Could you check a few things on this model? Use its own coordinates, in mm. A direction names the side the tool comes from. Give positions to 0.01 mm unless a question says otherwise; leave off trailing zeros. Write each loop counter-clockwise with the first axis right and the second up, starting at its lowest first coordinate (ties: lowest second). Pieces come first, ordered by that corner, then holes. Notation, with made-up numbers: M -10,-16.5 L 8,-16.5 A15 cw 8,7.5 Z; hole C 69.25,79.25 d7. An arc over 180 degrees is marked long. Answer as a JSON object with one key per item and string values. Group by question number.
```python
from build123d import *

# Parameters (mm, degrees)
F1_DEPTH    = 7.62
F2_T1_DEPTH = 231.4037837241


# Not quite as in the source:
# - a fillet or chamfer that OpenCascade refuses, or shapes differently, is made with other operations: its cross-section is extruded or revolved along the edge and cut away or added


with BuildPart() as f1:
    # F0 (on Top) → F1 (new body)
    with BuildSketch(Plane.XY):
        with BuildLine():
            ThreePointArc((64.7411976721, 47.7861853946), (-11.4588023279, 55.4061853946), (-87.6588023279, 47.7861853946))
            Line((-87.6588023279, 47.7861853946), (64.7411976721, 47.7861853946))
        make_face()
        with BuildLine():
            Line((-87.6588023279, -28.4138146054), (-87.6588023279, 47.7861853946))
            ThreePointArc((-87.6588023279, 47.7861853946), (-102.8988023279, 9.6861853946), (-87.6588023279, -28.4138146054))
        make_face()
        with BuildLine():
            Line((64.7411976721, 47.7861853946), (-87.6588023279, 47.7861853946))
            Line((-87.6588023279, 47.7861853946), (-87.6588023279, -28.4138146054))
            Line((-87.6588023279, -28.4138146054), (64.7411976721, -28.4138146054))
            ThreePointArc((64.7411976721, -28.4138146054), (58.4381171141, -26.858273051), (52.536175044, -24.1535339048))
            ThreePointArc((52.536175044, -24.1535339048), (51.7671122609, -23.7311786415), (51.0407896557, -23.2389419038))
            ThreePointArc((51.0407896557, -23.2389419038), (46.5861857996, -19.8140652327), (42.744152416, -15.7138146054))
            ThreePointArc((42.744152416, -15.7138146054), (46.5861857996, -11.6135639782), (51.0407896557, -8.188687307))
            ThreePointArc((51.0407896557, -8.188687307), (51.7671122609, -7.6964505693), (52.536175044, -7.2740953061))
            ThreePointArc((52.536175044, -7.2740953061), (58.4381171141, -4.5693561598), (64.7411976721, -3.0138146054))
            Line((64.7411976721, -3.0138146054), (64.7411976721, 22.3861853946))
            ThreePointArc((64.7411976721, 22.3861853946), (58.4381171141, 23.941726949), (52.536175044, 26.6464660952))
            ThreePointArc((52.536175044, 26.6464660952), (51.7671122609, 27.0688213585), (51.0407896557, 27.5610580962))
            ThreePointArc((51.0407896557, 27.5610580962), (46.5861857996, 30.9859347673), (42.744152416, 35.0861853946))
            ThreePointArc((42.744152416, 35.0861853946), (46.5861857996, 39.1864360218), (51.0407896557, 42.611312693))
            ThreePointArc((51.0407896557, 42.611312693), (51.7671122609, 43.1035494307), (52.536175044, 43.5259046939))
            ThreePointArc((52.536175044, 43.5259046939), (58.4381171141, 46.2306438402), (64.7411976721, 47.7861853946))
        make_face()
        with BuildLine():
            Line((64.7411976721, -28.4138146054), (-87.6588023279, -28.4138146054))
            ThreePointArc((-87.6588023279, -28.4138146054), (-11.4588023279, -36.0338146054), (64.7411976721, -28.4138146054))
        make_face()
        with BuildLine():
            ThreePointArc((51.0407896557, -23.2389419038), (49.0199759717, -21.171856557), (47.7230187251, -18.5883644093))
            Line((47.7230187251, -18.5883644093), (42.744152416, -15.7138146054))
            ThreePointArc((42.744152416, -15.7138146054), (46.5861857996, -19.8140652327), (51.0407896557, -23.2389419038))
        make_face()
        with BuildLine():
            Line((42.744152416, -15.7138146054), (47.7230187251, -18.5883644093))
            ThreePointArc((47.7230187251, -18.5883644093), (47.2726087596, -15.7138146054), (47.7230187251, -12.8392648016))
            Line((47.7230187251, -12.8392648016), (42.744152416, -15.7138146054))
        make_face()
        with BuildLine():
            ThreePointArc((51.0407896557, -8.188687307), (46.5861857996, -11.6135639782), (42.744152416, -15.7138146054))
            Line((42.744152416, -15.7138146054), (47.7230187251, -12.8392648016))
            ThreePointArc((47.7230187251, -12.8392648016), (49.0199759717, -10.2557726539), (51.0407896557, -8.188687307))
        make_face()
        with BuildLine():
            Line((42.744152416, 35.0861853946), (47.7230187251, 37.9607351984))
            ThreePointArc((47.7230187251, 37.9607351984), (49.0199759717, 40.5442273461), (51.0407896557, 42.611312693))
            ThreePointArc((51.0407896557, 42.611312693), (46.5861857996, 39.1864360218), (42.744152416, 35.0861853946))
        make_face()
        with BuildLine():
            ThreePointArc((47.7230187251, 32.2116355907), (47.2726087596, 35.0861853946), (47.7230187251, 37.9607351984))
            Line((47.7230187251, 37.9607351984), (42.744152416, 35.0861853946))
            Line((42.744152416, 35.0861853946), (47.7230187251, 32.2116355907))
        make_face()
        with BuildLine():
            Line((47.7230187251, 32.2116355907), (42.744152416, 35.0861853946))
            ThreePointArc((42.744152416, 35.0861853946), (46.5861857996, 30.9859347673), (51.0407896557, 27.5610580962))
            ThreePointArc((51.0407896557, 27.5610580962), (49.0199759717, 29.628143443), (47.7230187251, 32.2116355907))
        make_face()
    extrude(amount=F1_DEPTH)

    # F2: fillet of radius 43.18 on 2 edges, made by hand

    # F2_s2 → F2_t1 (cut)
    with BuildSketch(Plane.XY.offset(-111.891891862)):
        with BuildLine():
            ThreePointArc((-102.7512263975, 13.7215151075), (-93.3157996924, -16.5173565237), (-65.7822764709, -32.1801063989))
            ThreePointArc((-65.7822764709, -32.1801063989), (-76.7477031003, -30.4547410024), (-87.6588023279, -28.4138146054))
            ThreePointArc((-87.6588023279, -28.4138146054), (-99.6630733138, -8.9429787444), (-102.7512263975, 13.7215151075))
        make_face()
        with BuildLine():
            ThreePointArc((-65.7822764709, 51.552477188), (-93.3157996924, 35.8897273129), (-102.7512263975, 5.6508556816))
            ThreePointArc((-102.7512263975, 5.6508556816), (-99.6630733138, 28.3153495335), (-87.6588023279, 47.7861853946))
            ThreePointArc((-87.6588023279, 47.7861853946), (-76.7477031003, 49.8271117916), (-65.7822764709, 51.552477188))
        make_face()
    extrude(amount=F2_T1_DEPTH, mode=Mode.SUBTRACT)


solid = f1.part
```
1) If we section it at B-B, the plane x = 38: List the corners of the cut face in (y, z) for me, plus the area to 3 significant figures.
2) If we section it at C-C, the plane x = 12: List the corners of the cut face in (y, z) for me, plus the area to 3 significant figures.
3) If we section it at A-A, the plane z = 2.25: List the corners of the cut face in (x, y) for me.
4) For faces 1 (the cylindrical face through (58.35, 46.2, 3.76)), 2 (the cylindrical face through (0.56, 55.22, 3.76)), which set-ups out of +Z, -Z, +X, -X, +Y, -Y let a thin tool reach every point of the face, with its end or its side?
5) We'd pull the mould along Y, two halves only. Please class faces 3 (the cylindrical face through (-92.294, -17.74, 3.757)), 4 (the cylindrical face through (58.524, -26.888, 3.757)), 5 (the cylindrical face through (-91.73, 37.75, 3.76)): released by +Y, released by -Y, zero draft, split by the parting line, or undercut.
6) I'm going to push flat-ended pins straight in: pin 1 (1 mm diameter, centred on y = -1, z = 1, fed in from -X); pin 2 (6 mm diameter, centred on x = -66, y = -11.5, fed in from -Z); pin 3 (2 mm diameter, centred on y = 32, z = 3, fed in from -X). Where does each tip first touch, or does it pass through?
7) Please list where these lines run through material, in increasing order: line 1 along Y through (x, z) = (-91.5, 4.5); line 2 along X through (y, z) = (26, 2); line 3 along Y through (x, z) = (-60.5, 2.5). Write a range as from..to.
Taken from the geometry:
{
 "1": {"outline": "M -32.84,0 L 52.21,0 L 52.21,7.62 L -32.84,7.62 Z", "area": "648 mm²"},
 "2": {"outline": "M -35.32,0 L 54.69,0 L 54.69,7.62 L -35.32,7.62 Z", "area": "686 mm²"},
 "3": {"outline": "M -102.86,9.69 A43.18 ccw -65.78,-32.18 A384.81 ccw 64.74,-28.41 A34.63 cw 52.54,-24.15 A9.4 cw 52.54,-7.27 A34.63 cw 64.74,-3.01 L 64.74,22.39 A34.63 cw 52.54,26.65 A9.4 cw 52.54,43.53 A34.63 cw 64.74,47.79 A384.81 ccw -65.78,51.55 A43.18 ccw Z"},
 "4": {"face 1": "+Z, -Z, +X", "face 2": "+Z, -Z, +Y"},
 "5": {"face 3": "released by -Y", "face 4": "undercut", "face 5": "released by +Y"},
 "6": {"pin 1": "x = -101.42", "pin 2": "z = 0", "pin 3": "x = -96.73"},
 "7": {"line 1": "-18.63..38", "line 2": "-99.3..53.71", "line 3": "-32.9..52.27"}
}
